```python
from build123d import *

# Parameters (mm, degrees)
CYLINDER112_R             = 2.6
CYLINDER112_DEPTH         = 2
CYLINDER113_R             = 2.5
CYLINDER113_DEPTH         = 5
FUSION048_PLACEMENT_ANGLE = 90
CYLINDER109_R             = 2.6
CYLINDER109_DEPTH         = 2
CYLINDER108_R             = 2.5
CYLINDER108_DEPTH         = 5
FUSION043_PLACEMENT_ANGLE = 90
CYLINDER107_R             = 2.6
CYLINDER107_DEPTH         = 2
CYLINDER106_R             = 2.5
CYLINDER106_DEPTH         = 5
FUSION042_PLACEMENT_ANGLE = 90
CYLINDER103_R             = 2.6
CYLINDER103_DEPTH         = 2
CYLINDER102_R             = 2.5
CYLINDER102_DEPTH         = 5
FUSION040_PLACEMENT_ANGLE = 90
CYLINDER101_R             = 2.6
CYLINDER101_DEPTH         = 2
CYLINDER100_R             = 2.5
CYLINDER100_DEPTH         = 5
FUSION039_PLACEMENT_ANGLE = 90
CYLINDER099_R             = 6.5
CYLINDER099_DEPTH         = 130
CYLINDER110_R             = 2.6
CYLINDER110_DEPTH         = 2
CYLINDER111_R             = 2.5
CYLINDER111_DEPTH         = 5
FUSION046_PLACEMENT_ANGLE = 90
BOX028_W                  = 23
BOX028_H                  = 28
BOX028_DEPTH              = 4
BOX029_W                  = 7
BOX029_H                  = 28
BOX029_DEPTH              = 32
BOX027_W                  = 7
BOX027_H                  = 28
BOX027_DEPTH              = 32


with BuildPart() as cilindro112:
    # Cylinder112 → Cylinder112 (new body)
    with BuildSketch(Plane.XY.offset(5)):
        Circle(CYLINDER112_R)
    extrude(amount=CYLINDER112_DEPTH)


with BuildPart() as obj1:
    # Cylinder113 → Cylinder113 (new body)
    with BuildSketch(Plane.XY):
        Circle(CYLINDER113_R)
    extrude(amount=CYLINDER113_DEPTH)

    # Fusion048: union Cilindro112
    add(cilindro112.part)


with BuildPart() as obj1_1:
    # Fusion048 placement: moved
    add(obj1.part.moved(Location((0, 0, 16))).rotate(Axis((0, 0, 16), (0, 1, 0)), FUSION048_PLACEMENT_ANGLE))


with BuildPart() as cilindro109:
    # Cylinder109 → Cylinder109 (new body)
    with BuildSketch(Plane.XY.offset(5)):
        Circle(CYLINDER109_R)
    extrude(amount=CYLINDER109_DEPTH)


with BuildPart() as obj2:
    # Cylinder108 → Cylinder108 (new body)
    with BuildSketch(Plane.XY):
        Circle(CYLINDER108_R)
    extrude(amount=CYLINDER108_DEPTH)

    # Fusion043: union Cilindro109
    add(cilindro109.part)


with BuildPart() as obj2_1:
    # Fusion043 placement: moved
    add(obj2.part.moved(Location((23, 8, 16))).rotate(Axis((23, 8, 16), (0, -1, 0)), FUSION043_PLACEMENT_ANGLE))


with BuildPart() as cilindro107:
    # Cylinder107 → Cylinder107 (new body)
    with BuildSketch(Plane.XY.offset(5)):
        Circle(CYLINDER107_R)
    extrude(amount=CYLINDER107_DEPTH)


with BuildPart() as obj3:
    # Cylinder106 → Cylinder106 (new body)
    with BuildSketch(Plane.XY):
        Circle(CYLINDER106_R)
    extrude(amount=CYLINDER106_DEPTH)

    # Fusion042: union Cilindro107
    add(cilindro107.part)


with BuildPart() as obj3_1:
    # Fusion042 placement: moved
    add(obj3.part.moved(Location((23, -8, 16))).rotate(Axis((23, -8, 16), (0, -1, 0)), FUSION042_PLACEMENT_ANGLE))


with BuildPart() as cilindro103:
    # Cylinder103 → Cylinder103 (new body)
    with BuildSketch(Plane.XY.offset(5)):
        Circle(CYLINDER103_R)
    extrude(amount=CYLINDER103_DEPTH)


with BuildPart() as obj4:
    # Cylinder102 → Cylinder102 (new body)
    with BuildSketch(Plane.XY):
        Circle(CYLINDER102_R)
    extrude(amount=CYLINDER102_DEPTH)

    # Fusion040: union Cilindro103
    add(cilindro103.part)


with BuildPart() as obj4_1:
    # Fusion040 placement: moved
    add(obj4.part.moved(Location((0, -8, 16))).rotate(Axis((0, -8, 16), (0, 1, 0)), FUSION040_PLACEMENT_ANGLE))


with BuildPart() as cilindro101:
    # Cylinder101 → Cylinder101 (new body)
    with BuildSketch(Plane.XY.offset(5)):
        Circle(CYLINDER101_R)
    extrude(amount=CYLINDER101_DEPTH)


with BuildPart() as obj5:
    # Cylinder100 → Cylinder100 (new body)
    with BuildSketch(Plane.XY):
        Circle(CYLINDER100_R)
    extrude(amount=CYLINDER100_DEPTH)

    # Fusion039: union Cilindro101
    add(cilindro101.part)


with BuildPart() as obj5_1:
    # Fusion039 placement: moved
    add(obj5.part.moved(Location((0, 8, 16))).rotate(Axis((0, 8, 16), (0, 1, 0)), FUSION039_PLACEMENT_ANGLE))


with BuildPart() as cilindro099:
    # Cylinder099 → Cylinder099 (new body)
    with BuildSketch(Plane(origin=(-2, 0, 0), x_dir=(0, 0, -1), z_dir=(1, 0, 0))):
        Circle(CYLINDER099_R)
    extrude(amount=CYLINDER099_DEPTH)


with BuildPart() as cilindro110:
    # Cylinder110 → Cylinder110 (new body)
    with BuildSketch(Plane.XY.offset(5)):
        Circle(CYLINDER110_R)
    extrude(amount=CYLINDER110_DEPTH)


with BuildPart() as fusion047:
    # Cylinder111 → Cylinder111 (new body)
    with BuildSketch(Plane.XY):
        Circle(CYLINDER111_R)
    extrude(amount=CYLINDER111_DEPTH)

    # Fusion046: union Cilindro110
    add(cilindro110.part)


with BuildPart() as fusion047_1:
    # Fusion046 placement: moved
    add(fusion047.part.moved(Location((23, 0, 16))).rotate(Axis((23, 0, 16), (0, -1, 0)), FUSION046_PLACEMENT_ANGLE))

    # Fusion047: union obj2, obj3, obj4, obj5, Cilindro099
    add(obj2_1.part)
    add(obj3_1.part)
    add(obj4_1.part)
    add(obj5_1.part)
    add(cilindro099.part)


with BuildPart() as cubo025:
    # Box028 → Box028 (new body)
    with BuildSketch(Plane(origin=(0, -14, -11), x_dir=(1, 0, 0), z_dir=(0, 0, 1))):
        with Locations((11.5, 14)):
            Rectangle(BOX028_W, BOX028_H)
    extrude(amount=BOX028_DEPTH)


with BuildPart() as cubo026:
    # Box029 → Box029 (new body)
    with BuildSketch(Plane(origin=(16, -14, -11), x_dir=(1, 0, 0), z_dir=(0, 0, 1))):
        with Locations((3.5, 14)):
            Rectangle(BOX029_W, BOX029_H)
    extrude(amount=BOX029_DEPTH)


with BuildPart() as obj6:
    # Box027 → Box027 (new body)
    with BuildSketch(Plane(origin=(0, -14, -11), x_dir=(1, 0, 0), z_dir=(0, 0, 1))):
        with Locations((3.5, 14)):
            Rectangle(BOX027_W, BOX027_H)
    extrude(amount=BOX027_DEPTH)

    # Fusion045: union Cubo025, Cubo026
    add(cubo025.part)
    add(cubo026.part)

    # Cut054: cut Fusion047
    add(fusion047_1.part, mode=Mode.SUBTRACT)

    # Cut055: cut obj1
    add(obj1_1.part, mode=Mode.SUBTRACT)


solid = obj6.part
```
Source: CAD feature listing. Evaluate the final solid. Frame: model axes, mm. A direction names the side the tool comes from. Round coordinates to 2 decimals unless told otherwise and drop trailing zeros. Write each loop counter-clockwise with the first axis right and the second up, starting at its lowest first coordinate (ties: lowest second). Pieces come first, ordered by that corner, then holes. Notation, with made-up numbers: M 55.5,-7.75 L 70.5,-7.75 A23 cw 70.5,5.25 Z; hole C 16.25,35.25 d7. An arc over 180 degrees is marked long. Use CSV: the item, a comma, the result in double quotes. Start each with the question number.
Q1. Cut plane C-C on y = 8. Output: boundary loops of the cut face in (x, z), plus the area to 3 significant figures.
Q2. Line query: line 1 (Y direction, x = 21.7, z = 16); line 2 (Y direction, x = 17.1, z = 16); line 3 (X direction, y = -9.5, z = -1). Output: solid intervals per line, ascending. Write a range as from..to.
Q3. Cut plane D-D on x = 3.5. Output: boundary loops of the cut face in (y, z), plus the area to 3 significant figures.
Q4. Cut plane B-B on z = 0. Output: boundary loops of the cut face in (x, y), plus the area to 3 significant figures.
Q5. Cut plane A-A on z = 19. Output: boundary loops of the cut face in (x, y), plus the area to 3 significant figures.
Q6. Pull-direction query (Z, two-part tool) for faces 4 (the face through (2.5, 0.1, 18.5)), 5 (the face through (3, 0, 21)), 6 (the face through (23, 0, 8)); classes: +Z half, -Z half, draft (parallel to the pull), parting line (faces both ways), or undercut.
Q7. Access query for faces 1 (the face through (17, 7, 18.4)), 2 (the face through (16, 0, 7)), 3 (the face through (0, 0, 8)). Directions: +Z, -Z, +X, -X, +Y, -Y. A direction counts if a zero-diameter tool reaches every point of the face in a straight line with its end or side. Return the directions, or none.
Results found:
1,outline,"M 0,-11 L 23,-11 L 23,13.5 L 18,13.5 L 18,13.4 L 16,13.4 L 16,-7 L 7,-7 L 7,13.4 L 5,13.4 L 5,13.5 L 0,13.5 Z; M 0,18.5 L 5,18.5 L 5,18.6 L 7,18.6 L 7,21 L 0,21 Z; M 16,18.6 L 18,18.6 L 18,18.5 L 23,18.5 L 23,21 L 16,21 Z"
1,area,"413 mm^2"
2,line 1,"-14..-10.5, -5.5..-2.5, 2.5..5.5, 10.5..14"
2,line 2,"-14..-10.6, -5.4..-2.6, 2.6..5.4, 10.6..14"
2,line 3,"0..7, 16..23"
3,outline,"M -14,-11 L 14,-11 L 14,21 L -14,21 Z; hole C -8,16 d5; hole C 0,0 d13; hole C 0,16 d5; hole C 8,16 d5"
3,area,"704 mm^2"
4,outline,"M 0,-14 L 7,-14 L 7,-6.5 L 0,-6.5 Z; M 0,6.5 L 7,6.5 L 7,14 L 0,14 Z; M 16,-14 L 23,-14 L 23,-6.5 L 16,-6.5 Z; M 16,6.5 L 23,6.5 L 23,14 L 16,14 Z"
4,area,"210 mm^2"
5,outline,"M 0,-14 L 7,-14 L 7,14 L 0,14 Z; M 16,-14 L 23,-14 L 23,14 L 16,14 Z"
5,area,"392 mm^2"
6,face 4,"undercut"
6,face 5,"+Z half"
6,face 6,"draft"
7,face 1,"none"
7,face 2,"+Z, +Y, -Y"
7,face 3,"+Z, -Z, -X, +Y, -Y"
